```python
from build123d import *

# Parameters (mm, degrees)
F2_D     = 3
F2_DEPTH = 8.001
F3_D     = 3


with BuildPart() as f1:
    # F0 (on Front) → F1 (revolve)
    with BuildSketch(Plane.XZ):
        with BuildLine():
            Line((-23.4526408911, -24.7851572111), (-23.4526408911, 19.2148427889))
            Line((-23.4526408911, 19.2148427889), (-31.4526408911, 19.2148427889))
            Line((-31.4526408911, 19.2148427889), (-31.4526408911, 7.2148427889))
            Line((-31.4526408911, 7.2148427889), (-25.4526408911, 7.2148427889))
            Line((-25.4526408911, 7.2148427889), (-25.4526408911, -16.7851572111))
            Line((-25.4526408911, -16.7851572111), (-26.9526408911, -16.7851572111))
            ThreePointArc((-26.9526408911, -16.7851572111), (-27.3061942817, -16.9316038205), (-27.4526408911, -17.2851572111))
            Line((-27.4526408911, -17.2851572111), (-27.4526408911, -24.2851572111))
            ThreePointArc((-27.4526408911, -24.2851572111), (-27.3061942817, -24.6387106017), (-26.9526408911, -24.7851572111))
            Line((-26.9526408911, -24.7851572111), (-23.4526408911, -24.7851572111))
        make_face()
    revolve(axis=Axis((-23.4526408911, 0, -2.7851572111), (0, 0, -1)))

    # F2 (through all, one way)
    with BuildSketch(Plane(origin=(0, 0, 0), x_dir=(1, 0, 0), z_dir=(0, 1, 0))):
        with Locations((-23.4526408911, 20.7851572111)):
            Circle(F2_D / 2)
    extrude(amount=-F2_DEPTH, mode=Mode.SUBTRACT)

    # F3 (through all)
    with Locations(Plane.XZ):
        with Locations((-23.4526408911, -20.7851572111)):
            Hole(F3_D / 2)


solid = f1.part
```
Model file for the job. Use its own axes, mm. A direction names the side the tool comes from. Round coordinates to 2 decimals unless told otherwise and drop trailing zeros. Write each loop counter-clockwise with the first axis right and the second up, starting at its lowest first coordinate (ties: lowest second). Pieces come first, ordered by that corner, then holes. Notation, with made-up numbers: M 45.25,5.5 L 94.25,5.5 A27 ccw 94.25,22.5 Z; hole C -4.5,-35.75 d1. An arc over 180 degrees is marked long. Put each result on its own line as item: value.
Item 1: Cut at A-A (z = -20). List the corners of the cut face in (x, y), and give its area (3 significant figures).
Responses:
outline: M -24.73,-3.79 L -24.73,3.79 A4 ccw Z; M -22.17,-3.79 A4 ccw -22.17,3.79 Z
area: 30.2 mm²
Item 2: Cut at D-D (y = 5.5). List the corners of the cut face in (x, z).
Responses:
outline: M -29.26,7.21 L -17.64,7.21 L -17.64,19.21 L -29.26,19.21 Z
Item 3: Probe L1, parallel to Z at x = -24.75, y = -1.75; L2, parallel to Z at x = -24.5, y = -2; L3, parallel to Z at x = -21.75, y = 4. List the from-to ranges inside material, lowest first. Write a range as from..to.
Responses:
L1: -24.79..-21.54, -20.03..-16.79, 7.21..19.21
L2: -24.79..-21.86, -19.71..-16.79, 7.21..19.21
L3: 7.21..19.21
Item 4: Mould opens along Z. For faces 1 (the flat face through (-24, 0, 19.215)), 2 (the cylindrical face through (-17.104, -4.868, 13.131)), 3 (the flat face through (-22, -2, -16.785)) say: +Z half, -Z half, draft (parallel to the pull), parting line (faces both ways), or undercut.
Responses:
face 1: +Z half
face 2: draft
face 3: undercut
Item 5: Tool access for faces 4 (the cylindrical face through (-27.15, -1.53, -20.83)), 5 (the flat face through (-23, 0, -24.785)), 6 (the flat face through (-25, -2, 7.215)): list every direction of +Z, -Z, +X, -X, +Y, -Y with a clear straight run to the whole face (end or side of a thin tool).
Responses:
face 4: -Z
face 5: -Z, +X, -X, +Y, -Y
face 6: none
Item 6: Flat gauge pins, fed straight in: P1, Ø1, axis at y = -1, z = 0, coming from the -X side; P2, Ø2, axis at y = 5, z = -15, coming from the +X side; P3, Ø6, axis at x = -23.5, z = -18.5, coming from the -Y side; P4, Ø6, axis at x = -22.5, z = -12.5, coming from the +Y side. Where does each tip first touch, or does it go through?
Responses:
P1: x = -25.39
P2: through
P3: y = -4
P4: y = 2
Item 7: Cut at B-B (y = 2.75). State how many separate pieces and enclosed holes the cut face has, and give its area (3 significant figures).
Responses:
separate pieces: 2
enclosed holes: 1
area: 219 mm²
Item 8: Cut at C-C (z = 6). List the corners of the cut face in (x, y), and give its area (3 significant figures).
Responses:
outline: C -23.45,0 d4
area: 12.6 mm²
